The listing builds one solid part. Answer for the finished solid, in the listing's coordinates (mm). Coordinates: 2 decimals unless noted, no trailing zeros. Order: outer loops, then holes, each group sorted by start corner. A loop starts at its lowest first (then second) coordinate and runs counter-clockwise, first axis right, second up. Notation, with made-up numbers: M 48,24 L 94,24 A17 cw 94,49 Z; hole C -32,85.5 d6. An arc over 180 degrees is marked long. One line per item, written item: value. Start each with the question number.
Q1. Each of these flat-tipped pins is pushed along its axis until it touches: pin 1 Ø0.8 at (x, z) = (26.5, 1) entering from -Y; pin 2 Ø6 at (x, y) = (19.5, 57.5) entering from -Z; pin 3 Ø2 at (x, y) = (14, 53.5) entering from +Z; pin 4 Ø0.8 at (x, z) = (30.5, 0.5) entering from +Y. Where does it stop, or does it pass through?
Q2. Straight lines are drawn through the part: line 1 along Y through (x, z) = (-11, 1.2); line 2 along Z through (x, y) = (-0.5, 23.5); line 3 along Y through (x, z) = (27, 3.15). For each, find the intervals that lie inside material, in ascending order. Write a range as [from, to].
Q3. The part is cut by section A-A on y = 3. Give the vertices of the cut face in (x, z).
Q4. The part is cut by section C-C on y = 21.57. Give the vertices of the cut face in (x, z).
Q5. The part is cut by section B-B on x = -5. Give the vertices of the cut face in (y, z).
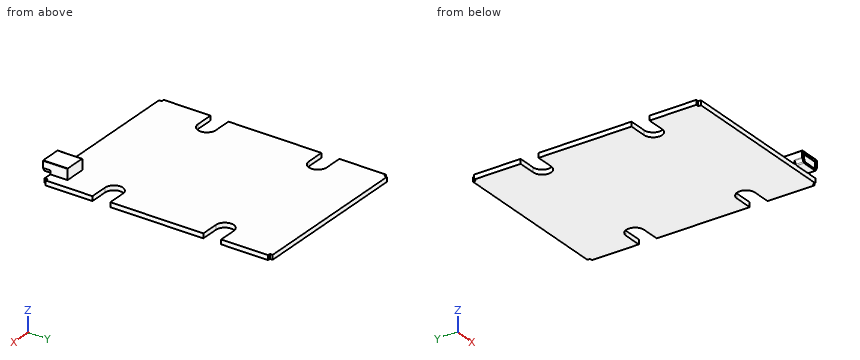
```python
from build123d import *

# Parameters (mm, degrees)
PAD_DEPTH    = 1.7
SKETCH005_W  = 7.77
SKETCH005_H  = 9.03
PAD006_DEPTH = 3.96
POCKET_DEPTH = 2.8
FILLET_R     = 0.2
FILLET001_R  = 0.2
FILLET007_R  = 0.2
FILLET008_R  = 0.5
FILLET009_R  = 0.5


with BuildPart() as part:
    # Sketch → Pad (new body)
    with BuildSketch(Plane.XY):
        with BuildLine():
            Line((0, 0), (30, 0))
            Line((30, 0), (30, 1))
            Line((30, 1), (31, 1))
            Line((31, 1), (31, 18.27))
            Line((31, 18.27), (24.4, 18.27))
            ThreePointArc((24.4, 24.87), (21.1, 21.57), (24.4, 18.27))
            Line((24.4, 24.87), (31, 24.87))
            Line((31, 24.87), (31, 59.13))
            Line((31, 59.13), (24.4, 59.13))
            ThreePointArc((24.4, 65.73), (21.1, 62.43), (24.4, 59.13))
            Line((24.4, 65.73), (31, 65.73))
            Line((31, 65.73), (31, 83))
            Line((30, 83), (31, 83))
            Line((30, 84), (30, 83))
            Line((30, 84), (0, 84))
            Line((0, 84), (-30, 84))
            Line((-30, 84), (-30, 83))
            Line((-30, 83), (-31, 83))
            Line((-31, 83), (-31, 65.73))
            Line((-31, 65.73), (-24.4, 65.73))
            ThreePointArc((-24.4, 59.13), (-21.1, 62.43), (-24.4, 65.73))
            Line((-24.4, 59.13), (-31, 59.13))
            Line((-31, 59.13), (-31, 24.87))
            Line((-31, 24.87), (-24.4, 24.87))
            ThreePointArc((-24.4, 18.27), (-21.1, 21.57), (-24.4, 24.87))
            Line((-24.4, 18.27), (-31, 18.27))
            Line((-31, 18.27), (-31, 1))
            Line((-31, 1), (-30, 1))
            Line((-30, 1), (-30, 0))
            Line((-30, 0), (0, 0))
        make_face()
    extrude(amount=PAD_DEPTH)

    # Sketch005 → Pad006 (new body)
    with BuildSketch(Plane.XY.offset(1.7)):
        with Locations((23.185, 1.815)):
            Rectangle(SKETCH005_W, SKETCH005_H)
    extrude(amount=PAD006_DEPTH)

    # Sketch011 → Pocket (cut)
    with BuildSketch(Plane.XZ.offset(2.7)):
        Polygon((19.3, 3.1), (19.3, 1.7), (20.05, 1.7), align=None)
        Polygon((27.07, 3.1), (27.07, 1.7), (26.32, 1.7), align=None)
        Polygon((19.6, 5.36), (26.77, 5.36), (26.77, 3.09), (26.186071, 2), (20.183929, 2), (19.6, 3.09), align=None)
        Polygon((20.3, 4.66), (20.3, 3.233333), (20.8, 2.3), (25.57, 2.3), (26.07, 3.233333), (26.07, 4.66), align=None, mode=Mode.SUBTRACT)
    extrude(amount=-POCKET_DEPTH, mode=Mode.SUBTRACT)

    # Fillet
    fillet_edges = [part.edges().sort_by_distance(p)[0] for p in [
        (27.07, 1.815, 5.66),
    ]]
    fillet(fillet_edges, radius=FILLET_R)

    # Fillet001
    fillet001_edges = [part.edges().sort_by_distance(p)[0] for p in [
        (19.3, 1.815, 5.66),
    ]]
    fillet(fillet001_edges, radius=FILLET001_R)

    # Fillet007
    fillet007_edges = [part.edges().sort_by_distance(p)[0] for p in [
        (27.07, -1.3, 3.1),
    ]]
    fillet(fillet007_edges, radius=FILLET007_R)

    # Fillet008
    fillet008_edges = [part.edges().sort_by_distance(p)[0] for p in [
        (26.32, -1.35, 1.7),
    ]]
    fillet(fillet008_edges, radius=FILLET008_R)

    # Fillet009
    fillet009_edges = [part.edges().sort_by_distance(p)[0] for p in [
        (19.3, -1.3, 3.1),
        (20.05, -1.35, 1.7),
    ]]
    fillet(fillet009_edges, radius=FILLET009_R)


solid = part.part
```
Output:
1. pin 1: stops at y = 0
1. pin 2: stops at z = 0
1. pin 3: stops at z = 1.7
1. pin 4: stops at y = 83
2. line 1: y = [0, 84]
2. line 2: z = [0, 1.7]
2. line 3: y = [-2.7, 6.33]
3. outline: M -31,0 L 31,0 L 31,1.7 L 27.07,1.7 L 27.07,5.46 A0.2 ccw 26.87,5.66 L 19.5,5.66 A0.2 ccw 19.3,5.46 L 19.3,1.7 L -31,1.7 Z
4. outline: M -21.1,0 L 21.1,0 L 21.1,1.7 L -21.1,1.7 Z
5. outline: M 0,0 L 84,0 L 84,1.7 L 0,1.7 Z
